Check sheet for the modelled part. Datum: model origin and axes. Units: mm. A direction names the side the tool comes from. Give positions to 0.01 mm unless a question says otherwise; leave off trailing zeros. Order: outer loops, then holes, each group sorted by start corner. A loop starts at its lowest first (then second) coordinate and runs counter-clockwise, first axis right, second up.
```python
from build123d import *

# Parameters (mm, degrees)
SKETCH_1_R        = 32.236701024
SKETCH_1_R_2      = 10.5
EXTRUDE_1_DEPTH   = 1.52
SKETCH_2_R        = 32.236701024
SKETCH_2_R_2      = 10.5
SKETCH_2_R_3      = 3.705
EXTRUDE_2_DEPTH   = 1.48
FILLET_1_R        = 1
SKETCH_3_R        = 5.705
SKETCH_3_R_2      = 3.705
EXTRUDE_1_2_DEPTH = 1.7


with BuildPart() as part:
    # 草图1 → Extrude 1 (new body)
    with BuildSketch(Plane.XY):
        Circle(SKETCH_1_R)
        with Locations((5.58185679, 19)):
            Circle(SKETCH_1_R_2, mode=Mode.SUBTRACT)
        with Locations((19.802957487, 0)):
            Circle(SKETCH_1_R_2, mode=Mode.SUBTRACT)
        with BuildLine():
            Line((-0.355524529, 3.687902833), (-16.411309781, 2.140078567))
            ThreePointArc((-16.411309781, 2.140078567), (-18.355, 0), (-16.411309781, -2.140078567))
            Line((-16.411309781, -2.140078567), (-0.355524529, -3.687902833))
            ThreePointArc((-0.355524529, -3.687902833), (3.705, 0), (-0.355524529, 3.687902833))
        make_face(mode=Mode.SUBTRACT)
    extrude(amount=-EXTRUDE_1_DEPTH)

    # 草图2 → 凸台-拉伸2 (add)
    with BuildSketch(Plane(origin=(0, 0, -1.52), x_dir=(-1, 0, 0), z_dir=(0, 0, -1))):
        Circle(SKETCH_2_R)
        with Locations((-5.58185679, 19)):
            Circle(SKETCH_2_R_2, mode=Mode.SUBTRACT)
        with Locations((-19.802957487, 0)):
            Circle(SKETCH_2_R_2, mode=Mode.SUBTRACT)
        Circle(SKETCH_2_R_3, mode=Mode.SUBTRACT)
    extrude(amount=EXTRUDE_2_DEPTH)

    # 圆角1
    fillet_1_edges = [part.edges().sort_by_distance(p)[0] for p in [
        (30.302957487, 0, -3),
        (16.08185679, 19, -3),
    ]]
    fillet(fillet_1_edges, radius=FILLET_1_R)

    # 草图3 → Extrude 1 2 (add)
    with BuildSketch(Plane(origin=(0, 0, -3), x_dir=(-1, 0, 0), z_dir=(0, 0, -1))):
        Circle(SKETCH_3_R)
        Circle(SKETCH_3_R_2, mode=Mode.SUBTRACT)
    extrude(amount=EXTRUDE_1_2_DEPTH)


solid = part.part
```
(1) Cross-section at D-D on y = 9.5. Count the separate pieces of the cut face and the enclosed holes in it, then the cut area to 3 significant figures.
Response values:
separate pieces: 3
enclosed holes: 0
area: 129 mm2
(2) Cross-section at C-C on x = -11. Enter the section's corners in (y, z), then the cut area to 3 significant figures.
Response values:
outline: (-30.3, -3) - (30.3, -3) - (30.3, 0) - (2.66, 0) - (2.66, -1.52) - (-2.66, -1.52) - (-2.66, 0) - (-30.3, 0) - close
area: 174 mm2
(3) Cross-section at B-B on y = 19. Enter the section's corners in (x, z).
Response values:
outline: (-26.04, -3) - (-5.92, -3) arc R1 ccw to (-4.92, -2) - (-4.92, 0) - (-26.04, 0) - close; (16.08, -2) arc R1 ccw to (17.08, -3) - (26.04, -3) - (26.04, 0) - (16.08, 0) - close
(4) Set-up check for faces 1 (the face through (0, -4, -4.7)), 2 (the face through (-8.271, 2.925, -0.749)): record each of +Z, -Z, +X, -X, +Y, -Y from which the full face is reachable in a straight line by a thin tool's end or side.
Response values:
face 1: -Z, +X, -X, +Y, -Y
face 2: +Z
(5) Gauge pin test, flat ends, axial feed: pin 1 Ø6 at (x, y) = (0, 0) entering from -Z; pin 2 Ø1 at (y, z) = (12, -2.5) entering from +X; pin 3 Ø1 at (x, z) = (-9.5, -2) entering from +Y; pin 4 Ø1.5 at (y, z) = (13.5, -2) entering from -X. Record the tip position at first contact, or that the pin passes through.
Response values:
pin 1: passes through
pin 2: stops at x = 30.12
pin 3: stops at y = 30.95
pin 4: stops at x = -29.61
(6) Release check for a two-part mould opening along X. For faces 3 (the face through (-8.496, -2.903, -0.749)), 4 (the face through (0, -7, 0)), 5 (the face through (4.53, -3.47, -3.84)) record: released by +X, released by -X, zero draft, split by the parting line, or undercut.
Response values:
face 3: undercut
face 4: zero draft
face 5: split by the parting line
(7) Material ranges on L1, parallel to Y at x = 0, z = -4.1 (3 decimals); L2, parallel to Y at x = 0, z = -1.2 (3 decimals); L3, parallel to Y at x = -4, z = -1.95, recorded low to high.
Response values:
L1: y = -5.705 to -3.705, 3.705 to 5.705
L2: y = -32.237 to -3.705, 3.705 to 10.107, 27.893 to 32.237
L3: y = -31.99 to 14.71, 23.29 to 31.99
(8) Cross-section at A-A on y = 0. Enter the section's corners in (x, z) (3 decimals).
Response values:
outline: (-32.237, -3) - (-5.705, -3) - (-5.705, -4.7) - (-3.705, -4.7) - (-3.705, -1.52) - (-18.355, -1.52) - (-18.355, 0) - (-32.237, 0) - close; (3.705, -4.7) - (5.705, -4.7) - (5.705, -3) - (8.303, -3) arc R1 ccw to (9.303, -2) - (9.303, 0) - (3.705, 0) - close; (30.303, -2) arc R1 ccw to (31.303, -3) - (32.237, -3) - (32.237, 0) - (30.303, 0) - close
